```python
from build123d import *

# Parameters (mm, degrees)
F0_W     = 45
F0_H     = 22
F1_DEPTH = 10
F2_W     = 15
F2_H     = 15
F3_DEPTH = 25
F4_SIZE  = 5
F5_R     = 4
F6_DEPTH = 15


with BuildPart() as f1:
    # F0 (on Front) → F1 (new body)
    with BuildSketch(Plane.XZ):
        with Locations((2.586208, 0)):
            Rectangle(F0_W, F0_H)
    extrude(amount=F1_DEPTH)

    # F2 (on face) → F3 (cut)
    with BuildSketch(Plane.XZ.offset(10)):
        with Locations((-4.913792, -3.5)):
            Rectangle(F2_W, F2_H)
        with Locations((10.086208, -3.5)):
            Rectangle(F2_W, F2_H)
    extrude(amount=-F3_DEPTH, mode=Mode.SUBTRACT)

    # F4
    f4_edges = [f1.edges().sort_by_distance(p)[0] for p in [
        (-19.913792, -5, 11),
        (25.086208, -5, 11),
    ]]
    chamfer(f4_edges, length=F4_SIZE)

    # F5 (on face) → F6 (join, through all)
    with BuildSketch(Plane(origin=(0, 0, 4), x_dir=(1, 0, 0), z_dir=(0, 0, -1))):
        with Locations((2.586208, 5)):
            Circle(F5_R)
    extrude(amount=F6_DEPTH)


solid = f1.part
```
The listing builds one solid part. Answer for the finished solid, in the listing's coordinates (mm). A direction names the side the tool comes from. Round coordinates to 2 decimals unless told otherwise and drop trailing zeros. Loops run counter-clockwise (first coordinate to the right, second up) from the corner with the lowest first, then second, coordinate; pieces in that order, holes last. Notation, with made-up numbers: (-26.75, 42.5) -> (28.25, 42.5) arc R28 ccw to (28.25, 80.5) -> close; hole circle Ø2 at (10.25, 89). An arc over 180 degrees is marked (long way). Use one line per item in the form item = value.
1. The part is cut by section C-C on x = 5. Determine the outline of the cut face in (y, z).
Answer key:
outline = (-10, 4) -> (-8.19, 4) -> (-8.19, -11) -> (-1.81, -11) -> (-1.81, 4) -> (0, 4) -> (0, 11) -> (-10, 11) -> close
2. The part is cut by section A-A on z = -5.75. Determine the outline of the cut face in (x, y).
Answer key:
outline = (-19.91, -10) -> (-12.41, -10) -> (-12.41, 0) -> (-19.91, 0) -> close; circle Ø8 at (2.59, -5); (17.59, -10) -> (25.09, -10) -> (25.09, 0) -> (17.59, 0) -> close
3. A tool of negligible diameter and unlimited length cuts with its end or side. For faces 1 (the flat face through (17.586, -5, -4)), 2 (the flat face through (2, -5, 11)), from which of +Z, -Z, +X, -X, +Y, -Y can it reach the whole face along a straight path? Write none if from no direction.
Answer key:
face_1 = -Z, +Y, -Y
face_2 = +Z, +X, -X, +Y, -Y
4. For a pull along X with two mould halves and no side action, classify faces 3 (the flat face through (3, -5, -11)), 4 (the flat face through (25.086, -5, -3)), 5 (the flat face through (-17.379, -4.93, 8.535)), 6 (the cylindrical face through (4.43, -1.45, -3.39)) as released by +X, released by -X, zero draft, split by the parting line, or undercut.
Answer key:
face_3 = zero draft
face_4 = released by +X
face_5 = released by -X
face_6 = undercut
5. The part is cut by section B-B on y = -5. Determine the outline of the cut face in (x, z), and give its area (3 significant figures).
Answer key:
outline = (-19.91, -11) -> (-12.41, -11) -> (-12.41, 4) -> (-1.41, 4) -> (-1.41, -11) -> (6.59, -11) -> (6.59, 4) -> (17.59, 4) -> (17.59, -11) -> (25.09, -11) -> (25.09, 6) -> (20.09, 11) -> (-14.91, 11) -> (-19.91, 6) -> close
area = 635 mm²
6. The part is cut by section D-D on y = -2.25. Determine the outline of the cut face in (x, z), and give its area (3 significant figures).
Answer key:
outline = (-19.91, -11) -> (-12.41, -11) -> (-12.41, 4) -> (-0.32, 4) -> (-0.32, -11) -> (5.49, -11) -> (5.49, 4) -> (17.59, 4) -> (17.59, -11) -> (25.09, -11) -> (25.09, 6) -> (20.09, 11) -> (-14.91, 11) -> (-19.91, 6) -> close
area = 602 mm²
7. Find the intervals of material crossed by probe 1 along X at (y, z) = (-9.5, -7); probe 2 along X at (y, z) = (-2.5, -8); probe 3 along X at (y, z) = (-3.75, 2), in increasing order. Write a range as [from, to].
Answer key:
probe_1 = [-19.91, -12.41], [17.59, 25.09]
probe_2 = [-19.91, -12.41], [-0.54, 5.71], [17.59, 25.09]
probe_3 = [-19.91, -12.41], [-1.21, 6.39], [17.59, 25.09]
